Can you work these out from the model? Positions are in its coordinate system, mm. A direction names the side the tool comes from. Coordinates: 2 decimals unless noted, no trailing zeros. Order: outer loops, then holes, each group sorted by start corner. A loop starts at its lowest first (then second) coordinate and runs counter-clockwise, first axis right, second up. Notation, with made-up numbers: (50, 54) -> (103, 54) arc R23 ccw to (103, 85) -> close; hole circle Ø5 at (-35.5, -12.75). An arc over 180 degrees is marked (long way). Use a Markdown table: item, result. Add a question column.
1. For pin 1 Ø4 at (x, z) = (7.5, 7.5) entering from +Y; pin 2 Ø2.5 at (x, z) = (-9, -0.5) entering from +Y; pin 3 Ø8 at (x, z) = (-10, 0) entering from -Y; pin 4 Ø10 at (x, z) = (1.5, -3) entering from -Y, each with a flat end and sliding along its axis, tell me the tip position at first contact or that it passes through.
2. Suppose I cut it at D-D, the plane x = 15.5. List the corners of the cut face in (y, z) for me, then the cut area to 3 significant figures.
3. Suppose I cut it at A-A, the plane z = 0. State how many separate pieces and enclosed holes the cut face has, then the cut area to 3 significant figures.
4. We'd pull the mould along X, two halves only. Please class faces 1 (the cylindrical face through (-12.44, 4.78, -0.54)), 2 (the flat face through (-17, -5, 0)), 3 (the flat face through (17, -5, 0)), 4 (the flat face through (14, -15, 0)): pulls with the +X half, pulls with the -X half, needs draft (parallel to the pull), parting line crosses it, or undercut.
5. For faces 5 (the cylindrical face through (13.578, -5.315, 0.596)), 6 (the flat face through (0, 0, 0)), 7 (the cylindrical face through (13.417, 5.986, 0.759)), which set-ups out of +Z, -Z, +X, -X, +Y, -Y let a thin tool reach every point of the face, with its end or its side?
6. Suppose I cut it at C-C, the plane y = -8. List the corners of the cut face in (x, z) for me.
7. Suppose I cut it at B-B, the plane y = -3.5. List the corners of the cut face in (x, z) for me, then the cut area to 3 significant figures.
8. If I drill on line 1 along X through (y, z) = (3.5, 0); line 2 along X through (y, z) = (-2.75, 4.75); line 3 along Y through (x, z) = (-12, 0), over which ranges is the centre line in solid material (lowest first)? Write a range as from..to.
```python
from build123d import *

# Parameters (mm, degrees)
SKETCH1_W            = 34
SKETCH1_H            = 20
BOSS_EXTRUDE1_DEPTH  = 5
SKETCH2_R            = 3.5
BOSS_EXTRUDE2_DEPTH  = 2
SKETCH3_R            = 2.5
CUT_EXTRUDE1_DEPTH   = 4.5
SKETCH4_W            = 6.75
SKETCH4_H            = 20
BOSS_EXTRUDE3_DEPTH  = 15
M5_CLEARANCE_HOLE1_D = 5.5


with BuildPart() as part:
    # Sketch1 → Boss-Extrude1 (new body)
    with BuildSketch(Plane(origin=(0, 0, 0), x_dir=(1, 0, 0), z_dir=(0, 1, 0))):
        Rectangle(SKETCH1_W, SKETCH1_H)
    extrude(amount=BOSS_EXTRUDE1_DEPTH)

    # Sketch2 → Boss-Extrude2 (add)
    with BuildSketch(Plane(origin=(0, 5, 0), x_dir=(1, 0, 0), z_dir=(0, 1, 0))):
        with Locations(Location((-10, 0, 0), (0, 0, 90))):
            Circle(SKETCH2_R)
        with Locations(Location((10, 0, 0), (0, 0, 90))):
            Circle(SKETCH2_R)
    extrude(amount=BOSS_EXTRUDE2_DEPTH)

    # Sketch3 → Cut-Extrude1 (cut)
    with BuildSketch(Plane(origin=(0, 7, 0), x_dir=(1, 0, 0), z_dir=(0, 1, 0))):
        with Locations(Location((-10, 0, 0), (0, 0, 270))):
            Circle(SKETCH3_R)
        with Locations(Location((10, 0, 0), (0, 0, 270))):
            Circle(SKETCH3_R)
    extrude(amount=-CUT_EXTRUDE1_DEPTH, mode=Mode.SUBTRACT)

    # Sketch4 → Boss-Extrude3 (add)
    with BuildSketch(Plane.XZ):
        with Locations((13.625, 0)):
            Rectangle(SKETCH4_W, SKETCH4_H)
        with Locations((-13.625, 0)):
            Rectangle(SKETCH4_W, SKETCH4_H)
    extrude(amount=BOSS_EXTRUDE3_DEPTH)

    # M5 Clearance Hole1 (through all)
    with Locations(Plane(origin=(17, -8, 0), x_dir=(0, 0, 1), z_dir=(1, 0, 0))):
        with Locations((0, 0)):
            Hole(M5_CLEARANCE_HOLE1_D / 2)


solid = part.part
```
Worked out:
| question | item | result |
|---|---|---|
| 1 | pin 1 | stops at y = 5 |
| 1 | pin 2 | stops at y = 2.5 |
| 1 | pin 3 | stops at y = -15 |
| 1 | pin 4 | stops at y = 0 |
| 2 | outline | (-15, -10) -> (5, -10) -> (5, 10) -> (-15, 10) -> close; hole circle Ø5.5 at (-8, 0) |
| 2 | area | 376 mm² |
| 3 | separate pieces | 3 |
| 3 | enclosed holes | 0 |
| 3 | area | 281 mm² |
| 4 | face 1 | undercut |
| 4 | face 2 | pulls with the -X half |
| 4 | face 3 | pulls with the +X half |
| 4 | face 4 | needs draft |
| 5 | face 5 | +X, -X |
| 5 | face 6 | +Z, -Z, -Y |
| 5 | face 7 | +Y |
| 6 | outline | (-17, -10) -> (-10.25, -10) -> (-10.25, -2.75) -> (-17, -2.75) -> close; (-17, 2.75) -> (-10.25, 2.75) -> (-10.25, 10) -> (-17, 10) -> close; (10.25, -10) -> (17, -10) -> (17, -2.75) -> (10.25, -2.75) -> close; (10.25, 2.75) -> (17, 2.75) -> (17, 10) -> (10.25, 10) -> close |
| 7 | outline | (-17, -10) -> (-10.25, -10) -> (-10.25, 10) -> (-17, 10) -> close; (10.25, -10) -> (17, -10) -> (17, 10) -> (10.25, 10) -> close |
| 7 | area | 270 mm² |
| 8 | line 1 | x = -17..-12.5, -7.5..7.5, 12.5..17 |
| 8 | line 2 | x = -17..-10.25, 10.25..17 |
| 8 | line 3 | y = -15..-10.75, -5.25..2.5 |
